Read the model definition and answer for the solid it produces. Units are mm, in the model's axes. A direction names the side the tool comes from. Give positions to 0.01 mm unless a question says otherwise; leave off trailing zeros. Write each loop counter-clockwise with the first axis right and the second up, starting at its lowest first coordinate (ties: lowest second). Pieces come first, ordered by that corner, then holes. Notation, with made-up numbers: (9.25, -15.5) -> (39.25, -15.5) arc R19 ccw to (39.25, -8.5) -> close; hole circle Ø9 at (44.25, -4.5). An arc over 180 degrees is marked (long way). Write item = value, one per line.
Autodesk Inventor part; units mm, degrees
ref_plane "YZ Plane" through (0, 0, 0) normal (1, 0, 0) x (0, 1, 0)
ref_plane "XZ Plane" through (0, 0, 0) normal (0, 1, 0) x (-1, 0, 0)
ref_plane "XY Plane" through (0, 0, 0) normal (0, 0, 1) x (1, 0, 0)
sketch "Sketch1" plane through (0, 0, 0) normal (0, 0, 1) x (1, 0, 0)
  line L0 (0, 0) -> (14.5304, 0)
  line L1 (-8.7854, 6.6412) -> (11.0866, 6.6412)
  line L2 (11.0866, 1.6412) -> (2.2606, 1.6412)
  line L3 (2.2606, 1.6412) -> (2.2606, -0.3588)
  line L4 (2.2606, -0.3588) -> (5.6256, -0.3588)
  line L5 (2.5721, -3.1588) -> (-3.1429, -3.1588)
  line L6 (-3.1429, -3.1588) -> (-5.8644, -1.1208)
  line L7 (-5.8644, -1.1208) -> (-5.8644, -0.3588)
  line L8 (-5.8644, -0.3588) -> (-2.4994, -0.3588)
  line L9 (-2.4994, -0.3588) -> (-2.4994, 1.6412)
  line L10 (-2.4994, 1.6412) -> (-8.7854, 1.6412)
  line L11 (-8.7854, 1.6412) -> (-8.7854, 6.6412)
  line L12 (5.6256, -0.3588) -> (5.6256, -1.1208)
  line L13 (5.6256, -1.1208) -> (2.5721, -3.1588)
  line L14 (11.0866, 6.6412) -> (5.0156, 6.6412)
  line L15 (5.0156, 1.6412) -> (11.0866, 1.6412)
  line L16 (11.0866, 6.6412) -> (11.0866, 1.6412)
  dimension "d2" = 5
  dimension "d3" = 2
  dimension "d6" = 11.49
  dimension "d7" = 2.921
  dimension "d9" = 5.6425
  dimension "d11" = 0.762
  dimension "d12" = 0.762
  dimension "d78" = 5.461
  dimension "d88" = 3.365
  dimension "d89" = 3.365
extrude "Extrusion1" add sketch "Sketch1" along normal blind 25.4
sketch "Sketch14" plane through (-8.7854, 1.6412, 0) normal (-1, 0, 0) x (0, 0, 1)
  line L0 (0, 0) -> (0, 5)
  line L1 (0, 0) -> (25.4, 0)
  line L2 (25.4, 5) -> (25.4, 0)
  line L3 (0, 5) -> (25.4, 5)
  line L4 (0, 5) -> (0, 0)
  line L5 (0, 0) -> (25.4, 0)
  line L6 (0, 5) -> (6.35, 5)
  line L7 (6.35, 5) -> (6.35, 0)
  line L8 (6.35, 0) -> (0, 0)
  line L9 (0, 0) -> (0, 5)
  point P0 (0, -1.6412)
  dimension "d161" = 6.35
extrude "Extrusion6" add sketch "Sketch14" along normal blind 9.525 contours L0 L3 L7 L1
sketch "Sketch17" plane through (-8.7854, 6.6412, 25.4) normal (0, 1, 0) x (1, 0, 0)
  line L0 (-9.525, 25.4) -> (19.872, 25.4)
  line L1 (-9.525, 19.05) -> (-9.525, 25.4)
  line L2 (0, 19.05) -> (-9.525, 19.05)
  line L3 (0, 19.05) -> (0, 0)
  line L4 (19.872, 0) -> (0, 0)
  line L5 (19.872, 25.4) -> (19.872, 0)
  line L6 (-9.525, 25.4) -> (19.872, 25.4)
  line L7 (19.872, 0) -> (0, 0)
  line L8 (19.872, 25.4) -> (13.522, 25.4)
  line L9 (13.522, 0) -> (19.872, 0)
  line L10 (19.872, 0) -> (19.872, 25.4)
  point P0 (8.7854, 25.4)
  dimension "d175" = 6.35
extrude "Extrusion9" add sketch "Sketch17" along normal blind 1.397
sketch "Sketch19" plane through (-8.7854, 1.6412, 25.4) normal (0, -1, 0) x (1, 0, 0)
  line L0 (6.286, -25.4) -> (-9.525, -25.4)
  line L1 (6.286, -25.4) -> (6.286, 0)
  line L2 (0, 0) -> (6.286, 0)
  line L3 (0, -19.05) -> (0, 0)
  line L4 (0, -19.05) -> (-9.525, -19.05)
  line L5 (-9.525, -25.4) -> (-9.525, -19.05)
  point P0 (8.7854, -25.4)
  point P1 (-4.7625, -22.225)
hole "Hole11" at (-13.5479, 1.6412, 3.175) direction (0, 1, 0) diameter 3.175 depth 25.4 tip angle 118
sketch "Sketch20" plane through (0, 0, 25.4) normal (0, 0, 1) x (1, 0, 0)
  line L0 (-8.7854, 1.6412) -> (-8.7854, 8.0382)
  line L1 (-8.7854, 1.6412) -> (-2.4994, 1.6412)
  line L2 (-2.4994, 1.6412) -> (-2.4994, -0.3588)
  line L3 (-2.4994, -0.3588) -> (-5.8644, -0.3588)
  line L4 (-5.8644, -0.3588) -> (-5.8644, -1.1208)
  line L5 (-5.8644, -1.1208) -> (-3.1429, -3.1588)
  line L6 (-3.1429, -3.1588) -> (2.5721, -3.1588)
  line L7 (2.5721, -3.1588) -> (5.6256, -1.1208)
  line L8 (5.6256, -1.1208) -> (5.6256, -0.3588)
  line L9 (5.6256, -0.3588) -> (2.2606, -0.3588)
  line L10 (2.2606, -0.3588) -> (2.2606, 1.6412)
  line L11 (2.2606, 1.6412) -> (11.0866, 1.6412)
  line L12 (11.0866, 1.6412) -> (11.0866, 8.0382)
  line L13 (-8.7854, 8.0382) -> (11.0866, 8.0382)
  point P0 (0, 0)
extrude "Extrusion10" add sketch "Sketch20" along normal blind 6.35
sketch "Sketch21" plane through (11.0866, 1.6412, 0) normal (1, 0, 0) x (0, 0, -1)
  line L0 (0, 6.397) -> (0, 0)
  line L1 (0, 6.397) -> (-31.75, 6.397)
  line L2 (-31.75, 0) -> (-31.75, 6.397)
  line L3 (0, 0) -> (-31.75, 0)
  point P0 (0, -1.6412)
  point P1 (-28.829, 3.222)
  point P2 (-9.271, 3.222)
  dimension "d199" = 31.75
  dimension "d200" = 19.558
  dimension "d201" = 9.271
  dimension "d202" = 3.175
  dimension "d203" = 3.175
hole "Hole12" at (11.0866, 4.8632, 28.829) at (11.0866, 4.8632, 9.271) direction (-1, 0, 0) diameter 3.556 depth 25.4 tip angle 118
equation "\"d9\" = -0.5 * d8 + 0.5 * d0"
equation "\"d12\" = d11"
properties part number "Sliderfor2020"
(1) Consider L1, parallel to Y at x = 4.75, z = 28.5; L2, parallel to Z at x = 7.25, y = 3.5; L3, parallel to Z at x = -6.25, y = 4. Determine where each line is inside the solid, lowest interval first.
Checks:
L1 = -1.71 to -0.36, 1.64 to 3.12, 6.61 to 8.04
L2 = 0 to 8.13, 10.41 to 27.69, 29.97 to 31.75
L3 = 0 to 7.72, 10.83 to 27.27, 30.38 to 31.75
(2) The part is cut by section A-A on y = 6. Count the separate pieces of the cut face and the enclosed holes in it, plus the area to 3 significant figures.
Checks:
separate_pieces = 3
enclosed_holes = 1
area = 575 mm²
(3) The part is cut by section B-B on x = -4.25. Determine the outline of the cut face in (y, z).
Checks:
outline = (-2.33, 0) -> (-0.36, 0) -> (-0.36, 31.75) -> (-2.33, 31.75) -> close; (1.64, 0) -> (8.04, 0) -> (8.04, 31.75) -> (1.64, 31.75) -> close; hole circle Ø3.56 at (4.86, 9.27); hole circle Ø3.56 at (4.86, 28.83)
(4) For a pull along X with two mould halves and no side action, classify faces 1 (the flat face through (4, -0.359, 16)), 2 (the cylindrical face through (-12.14, 4.88, 2.44)), 3 (the flat face through (2.261, 1, 16)) as released by +X, released by -X, zero draft, split by the parting line, or undercut.
Checks:
face_1 = zero draft
face_2 = undercut
face_3 = released by +X
(5) A tool of negligible diameter and unlimited length cuts with its end or side. For faces 4 (the flat face through (7, 1.641, 16)), 5 (the flat face through (-13, 5, 6.35)), 6 (the cylindrical face through (1.01, 5.95, 10.68)), 7 (the flat face through (-7, 1.641, 12)), 8 (the flat face through (-1, 8.038, 16)), from which of +Z, -Z, +X, -X, +Y, -Y can it reach the whole face along a straight path? Write none if from no direction.
Checks:
face_4 = +Z, -Z, +X
face_5 = +Z, -X, +Y, -Y
face_6 = +X, -X
face_7 = +Z, -Z, -X
face_8 = +Z, -Z, +X, -X, +Y
(6) The part is cut by section D-D on z = 22. Determine the outline of the cut face in (x, y).
Checks:
outline = (-8.79, 1.64) -> (-2.5, 1.64) -> (-2.5, -0.36) -> (-5.86, -0.36) -> (-5.86, -1.12) -> (-3.14, -3.16) -> (2.57, -3.16) -> (5.63, -1.12) -> (5.63, -0.36) -> (2.26, -0.36) -> (2.26, 1.64) -> (11.09, 1.64) -> (11.09, 8.04) -> (-8.79, 8.04) -> close
(7) Given P1, Ø1.9, axis at x = -13.55, z = 3.18, coming from the +Y side; P2, Ø1.5, axis at x = -9, z = 16.5, coming from the -Y side; P3, Ø1.5, axis at x = -15, y = 5, coming from the +Z side; P4, Ø17.5, axis at x = -12.5, z = 14, coming from the -Y side, each flat-ended and moving along its own axis, determine where each tip first touches the part or whether it passes through.
Checks:
P1 = through
P2 = 1.64
P3 = 6.35
P4 = -2.7
(8) The part is cut by section C-C on z = 29. Determine the outline of the cut face in (x, y).
Checks:
outline = (-8.79, 1.64) -> (-2.5, 1.64) -> (-2.5, -0.36) -> (-5.86, -0.36) -> (-5.86, -1.12) -> (-3.14, -3.16) -> (2.57, -3.16) -> (5.63, -1.12) -> (5.63, -0.36) -> (2.26, -0.36) -> (2.26, 1.64) -> (11.09, 1.64) -> (11.09, 3.09) -> (-8.79, 3.09) -> close; (-8.79, 6.63) -> (11.09, 6.63) -> (11.09, 8.04) -> (-8.79, 8.04) -> close
